Geometry: final body of the model. Coordinates: model frame, mm. Face numbers are marked on the shaded views. A direction names the side the tool comes from. Round coordinates to 2 decimals unless told otherwise and drop trailing zeros. Loops run counter-clockwise (first coordinate to the right, second up) from the corner with the lowest first, then second, coordinate; pieces in that order, holes last. Notation, with made-up numbers: (62.5, 12) - (117.5, 12) arc R17 ccw to (117.5, 41) - close; hole circle Ø3 at (-39, 86.5). An arc over 180 degrees is marked (long way). Answer as a JSON object with one key per item and string values. Group by question number.
Item 1: First-contact query: pin 1 (2 mm diameter, centred on x = 17, y = -7, fed in from +Z); pin 2 (3.5 mm diameter, centred on x = 16, y = -8, fed in from -Z); pin 3 (3.5 mm diameter, centred on x = 16, y = 8, fed in from +Z); pin 4 (2 mm diameter, centred on y = 9, z = 5, fed in from +X). Flat tips, straight axial feed; report the tip coordinate or a pass-through.
Item 2: Section D-D (x = 10.75). Return the cut outline in (y, z), plus the area to 3 significant figures.
Item 3: Section C-C (z = 6.75). Return the cut outline in (x, y).
Item 4: Section B-B (y = -3.75). Return the cut outline in (x, z), plus the area to 3 significant figures.
Item 5: Reachability of the marked faces 1, 2, 3 and 4 from +Z, -Z, +X, -X, +Y, -Y: full face, straight path, thin tool, end or side. Return the list, or none.
Item 6: Draft query along X for the marked faces 5, 6 and 7. Return one class per face: released by +X, released by -X, zero draft, split by the parting line, or undercut.
Item 7: Section A-A (z = 3). Return the cut outline in (x, y), plus the area to 3 significant figures.
Item 8: Line query: line 1 (Y direction, x = 16, z = 7.25); line 2 (Z direction, x = 14.75, y = 3.5); line 3 (X direction, y = -8, z = 0.8). Output: solid intervals per line, ascending.
Autodesk Inventor part; units mm, degrees
ref_plane "TopPlane" through (16.8435, -4.86, 8.0094) normal (0, 0, 1) x (1, 0, 0)
ref_plane "BottomPlane" through (16.7486, 4.86, 4.2094) normal (0, 0, -1) x (-1, 0, 0)
ref_plane "YZ Plane" through (0, 0, 0) normal (1, 0, 0) x (0, 1, 0)
sketch "Base" plane through (0, 0, 0) normal (0, 0, 1) x (1, 0, 0)
  circle A0 centre (16, -8) radius 2
  circle A1 centre (16, 8) radius 2
  circle A2 centre (16, -8) radius 3.5
  circle A3 centre (16, 8) radius 3.5
  point P0 (0, 0)
  dimension "d40" = 7
ref_plane "TopPlane" through (16.8435, -4.86, 8.0094) normal (0, 0, 1) x (1, 0, 0)
ref_plane "TopReferencePlane" through (16.8435, -4.86, 6.0094) normal (0, 0, 1) x (1, 0, 0)
extrude "BaseFeature" add sketch "Base" along normal up to surface (8.0094 mm away)
sketch "Cap" plane through (16, -8, 8.0094) normal (0, 0, 1) x (1, 0, 0)
  circle A0 centre (0, 0) radius 3.5 construction
  line L0 (3.5, 0) -> (6.5, 3.5753)
  line L1 (6.5, 3.5753) -> (6.5, 12.4247)
  line L2 (6.5, 12.4247) -> (3.5, 16)
  circle A1 centre (0, 16) radius 3.5 construction
  line L3 (-3.5, 0) -> (-3.5, 16) construction
  line L4 (-3.5, 8) -> (6.5, 8) construction
  circle A2 centre (0, 16) radius 3.5
  arc A3 (-3.5, 0) -> (3.5, 0) centre (0, 0) ccw
  arc A4 (3.5, 16) -> (-3.5, 16) centre (0, 16) ccw
  circle A5 centre (0, 0) radius 2
  circle A6 centre (0, 16) radius 2
  line L5 (0, 0) -> (0, 16) construction
  line L6 (-3.5, 0) -> (-6.5, 3.5753)
  line L7 (-6.5, 3.5753) -> (-6.5, 12.4247)
  line L8 (-6.5, 12.4247) -> (-3.5, 16)
  point P0 (-16, 8)
  point P1 (-3.5, 16)
  point P2 (-3.5, 0)
  dimension "d43" = 140
  dimension "d44" = 140
  dimension "d45" = 10
extrude "CapFeature" add sketch "Cap" along normal blind 3
ref_plane "BottomPlane" through (16.7486, 4.86, 4.2094) normal (0, 0, -1) x (-1, 0, 0)
ref_plane "BottomReferencePlane" through (16.7486, 4.86, 5.2094) normal (0, 0, -1) x (-1, 0, 0)
sketch "Bottom" plane through (16.7486, 4.86, 4.2094) normal (0, 0, -1) x (-1, 0, 0)
  arc A0 (4.2486, 3.14) -> (-2.7514, 3.14) centre (0.7486, 3.14) ccw
  line L0 (4.2486, 3.14) -> (7.2486, -0.4353)
  line L1 (7.2486, -0.4353) -> (7.2486, -9.2847)
  line L2 (7.2486, -9.2847) -> (4.2486, -12.86)
  arc A1 (-2.7514, -12.86) -> (4.2486, -12.86) centre (0.7486, -12.86) ccw
  line L3 (-2.7514, -12.86) -> (-5.7514, -9.2847)
  line L4 (-5.7514, -9.2847) -> (-5.7514, -0.4353)
  line L5 (-5.7514, -0.4353) -> (-2.7514, 3.14)
  circle A2 centre (0.7486, 3.14) radius 2
  circle A3 centre (0.7486, -12.86) radius 2
  point P0 (16.7486, -4.86)
extrude "BottomFeature" add sketch "Bottom" along normal blind 3 contours L0 L1 L2 A1 L3 L4 L5 A0 | A2 | A3
sketch "Sketch11" plane through (16, -8, 11.0094) normal (0, 0, 1) x (1, 0, 0)
  line L0 (-3, 10.1304) -> (3, 6.1304) construction
  line L1 (-3.8321, 8.8824) -> (2.1679, 4.8824)
  line L2 (3.8321, 7.3785) -> (-2.1679, 11.3785)
  arc A0 (-2.1679, 11.3785) -> (-3.8321, 8.8824) centre (-3, 10.1304) ccw
  arc A1 (2.1679, 4.8824) -> (3.8321, 7.3785) centre (3, 6.1304) ccw
  line L3 (-6.5, 12.4247) -> (-6.5, 3.5753)
  line L4 (6.5, 3.5753) -> (6.5, 12.4247)
  point P0 (-16, 8)
  point P1 (0, 8.1304)
  dimension "d52" = 3.5
  dimension "d53" = 3.5
  dimension "d54" = 1.5
extrude "Extrusion10" cut sketch "Sketch11" against normal through all
equation "\"d44\" = d43"
equation "\"d53\" = d52"
properties part number "PotentiometerBracket"
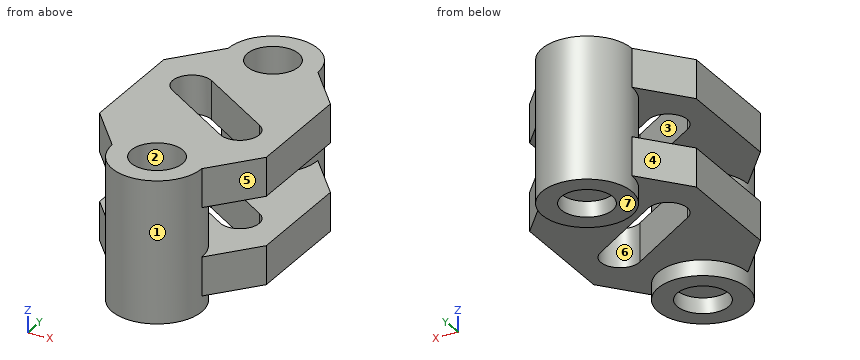
Values:
{
 "1": {"pin 1": "stops at z = 11.01", "pin 2": "stops at z = 1.21", "pin 3": "stops at z = 4.21", "pin 4": "stops at x = 19.5"},
 "2": {"outline": "(-5.91, 1.21) - (5.91, 1.21) - (5.91, 4.21) - (-5.91, 4.21) - close; (-5.91, 8.01) - (5.91, 8.01) - (5.91, 11.01) - (-5.91, 11.01) - close", "area": "71.0 mm^2"},
 "3": {"outline": "circle Ø7 at (16, -8); circle Ø7 at (16, 8); hole circle Ø4 at (16, -8); hole circle Ø4 at (16, 8)"},
 "4": {"outline": "(9.5, 1.21) - (22.5, 1.21) - (22.5, 4.21) - (9.5, 4.21) - close; (9.5, 8.01) - (22.5, 8.01) - (22.5, 11.01) - (9.5, 11.01) - close", "area": "78.0 mm^2"},
 "5": {"face 1": "none", "face 2": "+Z", "face 3": "+Z, -Z", "face 4": "+Z, -Z, -X, +Y"},
 "6": {"face 5": "released by +X", "face 6": "undercut", "face 7": "zero draft"},
 "7": {"outline": "(9.5, -4.42) - (12.5, -8) arc R3.5 ccw to (19.5, -8) - (22.5, -4.42) - (22.5, 4.42) - (19.5, 8) arc R3.5 ccw to (12.5, 8) - (9.5, 4.42) - close; hole (12.17, 0.88) - (18.17, -3.12) arc R1.5 ccw to (19.83, -0.62) - (13.83, 3.38) arc R1.5 ccw to start", "area": "196 mm^2"},
 "8": {"line 1": "y = -11.5 to -10, -6 to -4.5, 4.5 to 6, 10 to 11.5", "line 2": "z = 1.21 to 4.21, 8.01 to 11.01", "line 3": "x = 12.5 to 14, 18 to 19.5"}
}
